The figure shows three views and two pictorial views of one solid part (mm, origin at its lowest corner). Answer the questions. A direction names the side the tool comes from. Coordinates: 2 decimals unless noted, no trailing zeros. Loops run counter-clockwise (first coordinate to the right, second up) from the corner with the lowest first, then second, coordinate; pieces in that order, holes last. Notation, with made-up numbers: (22.5, 89.25) -> (49.5, 89.25) arc R26 cw to (49.5, 106.25) -> close; hole circle Ø11 at (53.25, 21.25). An arc over 180 degrees is marked (long way). Answer in a Markdown table with one row per item.
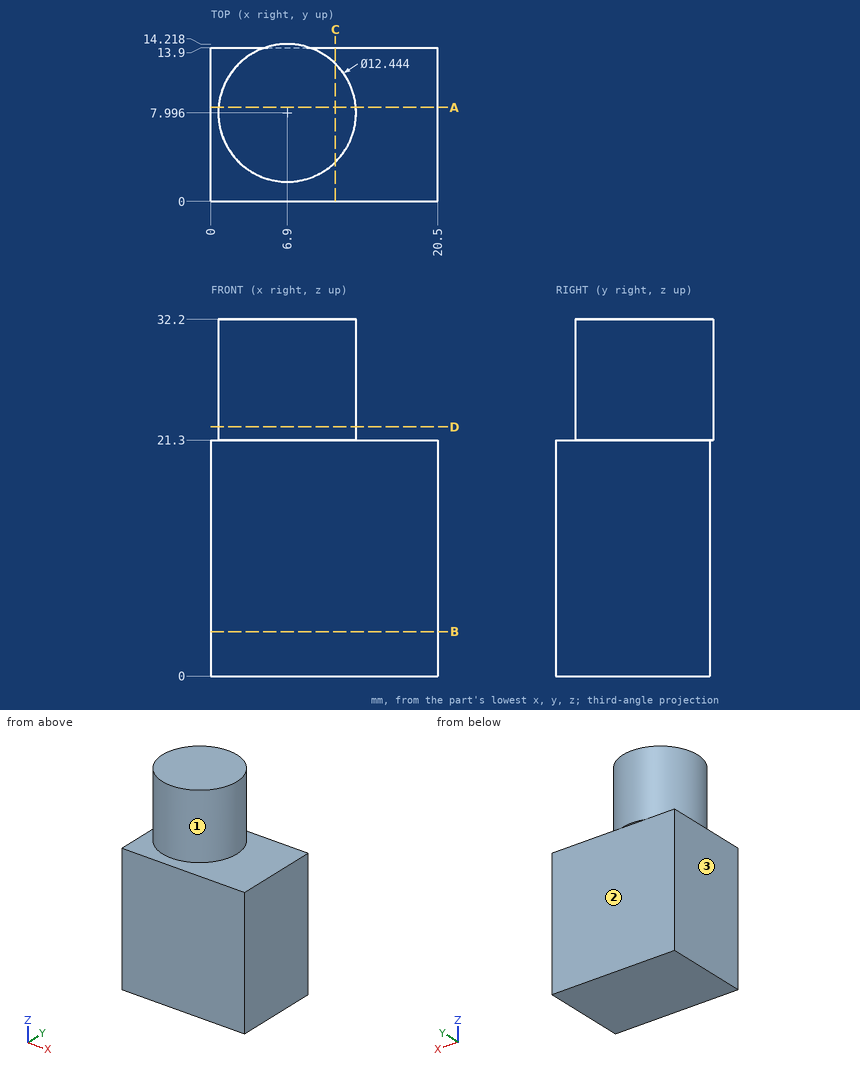
Item 1: Flat-ended cylindrical pins translate along their axes: pin 1 Ø3 at (x, z) = (2.5, 26) entering from -Y; pin 2 Ø10 at (x, z) = (10.5, 26.5) entering from +Y; pin 3 Ø6 at (x, z) = (14.5, 11) entering from +Y. Find the tip coordinate at first contact, or state that the pin passes through.
Findings below:
| item | result |
|---|---|
| pin 1 | stops at y = 2.49 |
| pin 2 | stops at y = 14.22 |
| pin 3 | stops at y = 13.9 |
Item 2: A cutting plane is placed at B-B, the plane z = 4. Determine the outline of the cut face in (x, y).
Findings below:
| item | result |
|---|---|
| outline | (0, 0) -> (20.5, 0) -> (20.5, 13.9) -> (0, 13.9) -> close |
Item 3: A cutting plane is placed at D-D, the plane z = 22.5. Determine the outline of the cut face in (x, y).
Findings below:
| item | result |
|---|---|
| outline | circle Ø12.44 at (6.9, 8) |
Item 4: Find the intervals of material crossed by probe 1 along Z at (x, y) = (14.25, 8.25); probe 2 along Y at (x, z) = (3.5, 20.5); probe 3 along X at (y, z) = (11.5, 30.5), in increasing order.
Findings below:
| item | result |
|---|---|
| probe 1 | z = 0 to 21.3 |
| probe 2 | y = 0 to 13.9 |
| probe 3 | x = 1.76 to 12.04 |
Item 5: A cutting plane is placed at C-C, the plane x = 11.25. Determine the outline of the cut face in (y, z) (1 decimal), plus the area to 3 significant figures.
Findings below:
| item | result |
|---|---|
| outline | (0, 0) -> (13.9, 0) -> (13.9, 21.3) -> (12.4, 21.3) -> (12.4, 32.2) -> (3.5, 32.2) -> (3.5, 21.3) -> (0, 21.3) -> close |
| area | 393 mm2 |
Item 6: A tool of negligible diameter and unlimited length cuts with its end or side. For the marked faces 1, 2 and 3, from which of +Z, -Z, +X, -X, +Y, -Y can it reach the whole face along a straight path? Write none if from no direction.
Findings below:
| item | result |
|---|---|
| face 1 | +Z |
| face 2 | -Z, +X, -X, +Y |
| face 3 | +Z, -Z, -X, +Y, -Y |
Item 7: A cutting plane is placed at A-A, the plane y = 8.5. Determine the outline of the cut face in (x, z).
Findings below:
| item | result |
|---|---|
| outline | (0, 0) -> (20.5, 0) -> (20.5, 21.3) -> (13.1, 21.3) -> (13.1, 32.2) -> (0.7, 32.2) -> (0.7, 21.3) -> (0, 21.3) -> close |
